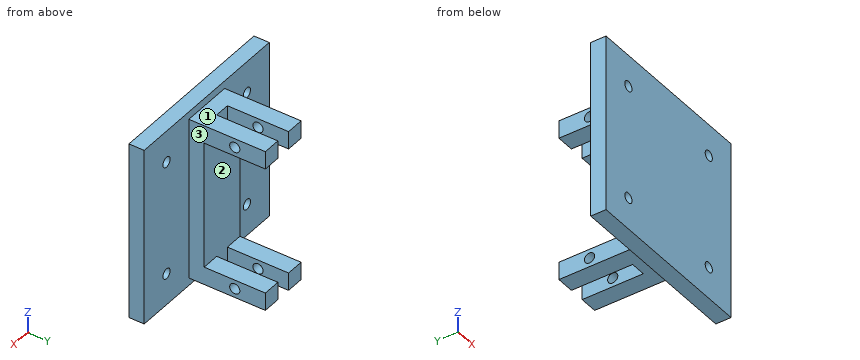
Autodesk Inventor part; units mm, degrees
ref_plane "YZ Plane" through (0, 0, 0) normal (1, 0, 0) x (0, 1, 0)
ref_plane "XZ Plane" through (0, 0, 0) normal (0, 1, 0) x (-1, 0, 0)
ref_plane "XY Plane" through (0, 0, 0) normal (0, 0, 1) x (1, 0, 0)
sketch "Sketch1" plane through (0, 0, 0) normal (0, 1, 0) x (-1, 0, 0)
  circle A0 centre (11.25, 11.25) radius 1
  circle A1 centre (11.25, -11.25) radius 1
  circle A2 centre (-11.25, 11.25) radius 1
  circle A3 centre (-11.25, -11.25) radius 1
  line L0 (-17.5, 17.5) -> (17.5, 17.5)
  line L1 (17.5, 17.5) -> (17.5, -17.5)
  line L2 (17.5, -17.5) -> (-17.5, -17.5)
  line L3 (-17.5, -17.5) -> (-17.5, 17.5)
  line L4 (-5, 16) -> (5, 16)
  line L5 (5, 16) -> (5, -16)
  line L6 (5, -16) -> (-5, -16)
  line L7 (-5, -16) -> (-5, 16)
  line L8 (-5, -16) -> (-1.5, -16)
  line L9 (-1.5, -16) -> (-1.5, -12.5)
  line L10 (-1.5, -12.5) -> (-5, -12.5)
  line L11 (-5, -12.5) -> (-5, -16)
  line L12 (5, -16) -> (1.5, -16)
  line L13 (1.5, -16) -> (1.5, -12.5)
  line L14 (1.5, -12.5) -> (5, -12.5)
  line L15 (5, -12.5) -> (5, -16)
  line L16 (-5, 16) -> (-1.5, 16)
  line L17 (-1.5, 16) -> (-1.5, 12.5)
  line L18 (-1.5, 12.5) -> (-5, 12.5)
  line L19 (-5, 12.5) -> (-5, 16)
  line L20 (5, 16) -> (1.5, 16)
  line L21 (1.5, 16) -> (1.5, 12.5)
  line L22 (1.5, 12.5) -> (5, 12.5)
  line L23 (5, 12.5) -> (5, 16)
  point P0 (0, 0)
extrude "Extrusion1" add sketch "Sketch1" along normal blind 18 contours L4 L17 L18 L7 | L4 L5 L22 L21 | L10 L9 L6 L7 | L5 L6 L13 L14
extrude "Extrusion2" add sketch "Sketch1" along normal blind 6 contours L4 L21 L22 L5 L14 L13 L6 L9 L10 L7 L18 L17
extrude "Extrusion3" add sketch "Sketch1" along normal blind 3
sketch "Sketch2" plane through (5, 18, -12.5) normal (1, 0, 0) x (0, 0, -1)
  line L0 (-28.5, -12) -> (-25, -12)
  line L1 (3.5, -12) -> (0, -12)
  circle A0 centre (1.75, -6) radius 1
  circle A1 centre (-26.75, -6) radius 1
  point P0 (-12.5, -18)
extrude "Extrusion4" cut sketch "Sketch2" against normal blind 3.5
sketch "Sketch3" plane through (-5, 18, 12.5) normal (-1, 0, 0) x (0, 0, 1)
  circle A0 centre (-26.75, -6) radius 1
  circle A1 centre (-26.75, -6) radius 1
  circle A2 centre (1.75, -6) radius 1
  circle A3 centre (1.75, -6) radius 1
  point P0 (-12.5, -18)
extrude "Extrusion5" cut sketch "Sketch3" against normal blind 3.5 contours A0
extrude "Extrusion6" cut sketch "Sketch3" against normal blind 3.5 contours A2
properties part number "camera_plate"
Can you work these out from the model? Positions are in its coordinate system, mm. Face numbers are marked on the shaded views. Give positions to 0.01 mm unless a question says otherwise; leave off trailing zeros. Loops run counter-clockwise (first coordinate to the right, second up) from the corner with the lowest first, then second, coordinate; pieces in that order, holes last. Notation, with made-up numbers: M -2.75,18 L 16.25,18 A26 ccw 16.25,36 Z; hole C 52,42 d7. An arc over 180 degrees is marked long. Use CSV: the item, a comma, the result in double quotes. Start each with the question number.
1. If I drill on L1, parallel to Z at x = 11.25, y = 2.1; L2, parallel to X at y = 7.75, z = -13; L3, parallel to Y at x = 2.4, z = 14.25, over which ranges is the centre line in solid material (lowest first)?
2. If we mould it in two halves opening along Z, with no side actions, what happens to the marked faces 1, 2 and 3? For each: released by +Z, released by -Z, zero draft, split by the parting line, or undercut.
3. For P1, Ø2.5, axis at x = 11.25, z = 11.25, coming from the +Y side; P2, Ø1.8, axis at y = 12, z = 14.25, coming from the -X side; P3, Ø4, axis at x = 4, y = 8, coming from the -Z side; P4, Ø4, axis at x = -3.5, y = 11, coming from the +Z side, each with a flat end and sliding along its axis, tell me the tip position at first contact or that it passes through.
4. Imagine slicing it at A-A, the plane y = 16.75. Write out the boundary of the cut face in (x, z).
5. Imagine slicing it at B-B, the plane z = -14.25. Write out the boundary of the cut face in (x, y), plus the area to 3 significant figures.
6. Imagine slicing it at D-D, the plane x = 11.25. Write out the boundary of the cut face in (y, z).
7. Imagine slicing it at C-C, the plane y = 12. Count the separate pieces of the cut face and the enclosed holes in it, plus the area to 3 significant figures.
Response values:
1,L1,"-17.5 to -12.25, -10.25 to 10.25, 12.25 to 17.5"
1,L2,"-5 to -1.5, 1.5 to 5"
1,L3,"0 to 11, 13 to 18"
2,face 1,"released by +Z"
2,face 2,"undercut"
2,face 3,"zero draft"
3,P1,"y = 3"
3,P2,"through"
3,P3,"z = -16"
3,P4,"z = 16"
4,outline,"M -5,-16 L -1.5,-16 L -1.5,-12.5 L -5,-12.5 Z; M -5,12.5 L -1.5,12.5 L -1.5,16 L -5,16 Z; M 1.5,-16 L 5,-16 L 5,-12.5 L 1.5,-12.5 Z; M 1.5,12.5 L 5,12.5 L 5,16 L 1.5,16 Z"
5,outline,"M -17.5,0 L 17.5,0 L 17.5,3 L 5,3 L 5,11 L 1.5,11 L 1.5,6 L -1.5,6 L -1.5,11 L -5,11 L -5,3 L -17.5,3 Z; M -5,13 L -1.5,13 L -1.5,18 L -5,18 Z; M 1.5,13 L 5,13 L 5,18 L 1.5,18 Z"
5,area,"205 mm^2"
6,outline,"M 0,-17.5 L 3,-17.5 L 3,-12.25 L 0,-12.25 Z; M 0,-10.25 L 3,-10.25 L 3,10.25 L 0,10.25 Z; M 0,12.25 L 3,12.25 L 3,17.5 L 0,17.5 Z"
7,separate pieces,"8"
7,enclosed holes,"0"
7,area,"21.0 mm^2"
